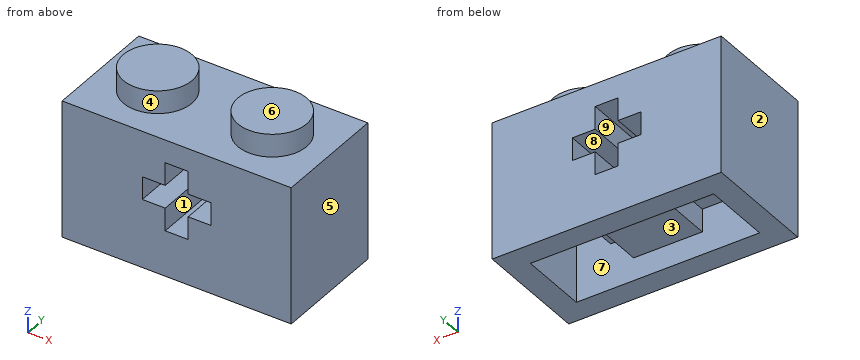
from build123d import *

# Parameters (mm, degrees)
F0_W        = 15.875
F0_H        = 9.525
F1_DEPTH    = 7.9375
F2_T        = 1.5875
F2_T3_DEPTH = 11.1125
F3_R        = 2.38125
F4_DEPTH    = 1.5875


# Not quite as in the source:
# - a shell that OpenCascade refuses in one call is made with other operations: the cavity is built on its own and cut out


with BuildPart() as f1:
    # F0 (on Front) → F1 (new body)
    with BuildSketch(Plane.XZ):
        Rectangle(F0_W, F0_H)
        Polygon((-0.79375, 1.5875), (-0.79375, 3.175), (0.79375, 3.175), (0.79375, 1.5875), (2.38125, 1.5875), (2.38125, 0), (0.79375, 0), (0.79375, -1.5875), (-0.79375, -1.5875), (-0.79375, 0), (-2.38125, 0), (-2.38125, 1.5875), align=None, mode=Mode.SUBTRACT)
    extrude(amount=F1_DEPTH)

    # F2: shell of thickness 1.5875, made by hand


with BuildPart() as f2_core1:
    # F2_t2: copy of F1
    add(f1.part)

    # the walls: a layer under each face that stays
    f2_faces = [f2_core1.faces().sort_by_distance(p)[0] for p in [
        (0, -3.96875, 4.7625),
        (-7.9375, -3.96875, 0),
        (7.9375, -3.96875, 0),
        (-0.79375, -3.96875, -0.79375),
        (-1.5875, -3.96875, 0),
        (-2.38125, -3.96875, 0.79375),
        (-1.5875, -3.96875, 1.5875),
        (-0.79375, -3.96875, 2.38125),
        (0, -3.96875, 3.175),
        (0.79375, -3.96875, 2.38125),
        (1.5875, -3.96875, 1.5875),
        (2.38125, -3.96875, 0.79375),
        (1.5875, -3.96875, 0),
        (0.79375, -3.96875, -0.79375),
        (0, -3.96875, -1.5875),
        (-5.2916666667, 0, -3.175),
        (-5.2916666667, -7.9375, -3.175),
    ]]
    thicken(f2_faces, amount=-F2_T, mode=Mode.SUBTRACT)

    # F2_s4 → F2_t3 (cut)
    with BuildSketch(Plane.XZ.offset(-1.5875)):
        Polygon((-0.777875, -1.571625), (-2.38125, -1.5875), (-2.38125, -3.175), (-0.79375, -3.175), align=None)
        Polygon((-2.365375, 0.015875), (-2.38125, -1.5875), (-3.96875, -1.5875), (-3.96875, 0), align=None)
        Polygon((-2.365375, 1.571625), (-3.96875, 1.5875), (-3.96875, 3.175), (-2.38125, 3.175), align=None)
        Polygon((-0.777875, 3.159125), (-2.38125, 3.175), (-2.38125, 4.7625), (-0.79375, 4.7625), align=None)
        Polygon((0.777875, 3.159125), (0.79375, 4.7625), (2.38125, 4.7625), (2.38125, 3.175), align=None)
        Polygon((2.365375, 1.571625), (2.38125, 3.175), (3.96875, 3.175), (3.96875, 1.5875), align=None)
        Polygon((2.365375, 0.015875), (3.96875, 0), (3.96875, -1.5875), (2.38125, -1.5875), align=None)
        Polygon((0.777875, -1.571625), (2.38125, -1.5875), (2.38125, -3.175), (0.79375, -3.175), align=None)
    extrude(amount=F2_T3_DEPTH, mode=Mode.SUBTRACT)


with BuildPart() as f1_1:
    add(f1.part)

    # what is left inside the walls is the cavity
    f2_cavity = [f2_core1.part.solids().sort_by_distance(p)[0] for p in [
        (0, -4.7625, -4.746625),
    ]]
    add(f2_cavity, mode=Mode.SUBTRACT)

    # F3 (on face) → F4 (join)
    with BuildSketch(Plane.XY.offset(4.7625)):
        with Locations((-3.96875, -3.96875)):
            Circle(F3_R)
        with Locations((3.96875, -3.96875)):
            Circle(F3_R)
    extrude(amount=F4_DEPTH)


solid = f1_1.part
Check sheet for the modelled part. Datum: model origin and axes. Units: mm. Face numbers are marked on the shaded views. A direction names the side the tool comes from. Coordinates: 2 decimals unless noted, no trailing zeros. Loops run counter-clockwise (first coordinate to the right, second up) from the corner with the lowest first, then second, coordinate; pieces in that order, holes last. Notation, with made-up numbers: (68, -36) -> (126, -36) arc R20 ccw to (126, -23) -> close; hole circle Ø11 at (42.5, 57.25). An arc over 180 degrees is marked (long way). Write item = value, one per line. Start each with the question number.
1. Section check C-C on y = -1. Record the cut outline in (x, z) (1 decimal).
2. Tool access check on the marked faces 1, 2, 3, 4 and 5. Record the directions out of +Z, -Z, +X, -X, +Y, -Y that give a thin tool (end or side, any length) a straight path to the whole face; none if there is none.
3. Section check D-D on z = -3.5. Record the cut outline in (x, y), then the cut area to 3 significant figures.
4. Depth check by flat-ended pin: P1, Ø1.7, axis at x = 0, y = -2.5, coming from the +Z side; P2, Ø2.5, axis at x = -5.5, y = -5, coming from the -Z side; P3, Ø1.3, axis at x = -1.5, y = -2.5, coming from the -Z side (3 decimals); P4, Ø0.7, axis at x = 5, y = -3.5, coming from the -Z side (3 decimals). Enter the tip coordinate at first touch or a pass-through.
5. Material ranges on line 1 (X direction, y = -4, z = 3); line 2 (Y direction, x = 3, z = -3.25), recorded low to high.
6. Section check B-B on z = -2.25. Record the cut outline in (x, y).
7. Draft check along Z on the marked faces 6, 7, 8 and 9. Enter one of: released by +Z, released by -Z, zero draft, split by the parting line, or undercut.
Responses:
q1.outline = (-7.9, -4.8) -> (7.9, -4.8) -> (7.9, 4.8) -> (-7.9, 4.8) -> close; hole (-2.4, 0) -> (-0.8, 0) -> (-0.8, -1.6) -> (0.8, -1.6) -> (0.8, 0) -> (2.4, 0) -> (2.4, 1.6) -> (0.8, 1.6) -> (0.8, 3.2) -> (-0.8, 3.2) -> (-0.8, 1.6) -> (-2.4, 1.6) -> close
q2.face_1 = +Y, -Y
q2.face_2 = +Z, -Z, -X, +Y, -Y
q2.face_3 = -Z
q2.face_4 = +Z
q2.face_5 = +Z, -Z, +X, +Y, -Y
q3.outline = (-7.94, -7.94) -> (7.94, -7.94) -> (7.94, 0) -> (-7.94, 0) -> close; hole (-6.35, -6.35) -> (6.35, -6.35) -> (6.35, -1.59) -> (-6.35, -1.59) -> close
q3.area = 65.5 mm2
q4.P1 = 4.76
q4.P2 = -4.76
q4.P3 = -3.175
q4.P4 = 3.175
q5.line_1 = -7.94 to -6.35, -3.97 to -0.79, 0.79 to 3.97, 6.35 to 7.94
q5.line_2 = -7.94 to -6.35, -1.59 to 0
q6.outline = (-7.94, -7.94) -> (7.94, -7.94) -> (7.94, 0) -> (-7.94, 0) -> close; hole (-6.35, -6.35) -> (-2.38, -6.35) -> (-2.38, -1.59) -> (-6.35, -1.59) -> close; hole (2.38, -6.35) -> (6.35, -6.35) -> (6.35, -1.59) -> (2.38, -1.59) -> close
q7.face_6 = released by +Z
q7.face_7 = zero draft
q7.face_8 = undercut
q7.face_9 = undercut
